Design review of the part built by this model. Coordinates are the model's own, in mm. Face numbers are marked on the shaded views. Coordinates: 2 decimals unless noted, no trailing zeros. Write each loop counter-clockwise with the first axis right and the second up, starting at its lowest first coordinate (ties: lowest second). Pieces come first, ordered by that corner, then holes. Notation, with made-up numbers: (-9, 72.25) - (11, 72.25) arc R14 cw to (11, 79.25) - close; hole circle Ø3 at (10, 35). An arc over 180 degrees is marked (long way). Answer as a JSON object with one key per item and string values.
```python
from build123d import *

# Parameters (mm, degrees)
EXTRUDE1_DEPTH = 2.286


with BuildPart() as part:
    # Sketch1 → Extrude1 (new body)
    with BuildSketch(Plane(origin=(0, 0, 0), x_dir=(1, 0, 0), z_dir=(0, 1, 0))):
        with BuildLine():
            Line((-35.587506478, 37.75591133), (35.587506478, 37.75591133))
            ThreePointArc((35.587506478, 37.75591133), (37.512064818, 37.331110288), (39.078987817, 36.135646762))
            Line((39.078987817, 36.135646762), (51.39211015, 21.570982059))
            ThreePointArc((51.39211015, 21.570982059), (52.406608959, 19.393408694), (52.177078973, 17.002101608))
            Line((52.177078973, 17.002101608), (36.497605157, -24.461395817))
            ThreePointArc((36.497605157, -24.461395817), (34.820154512, -26.605684768), (32.221154995, -27.416250797))
            Line((32.221154995, -27.416250797), (-32.221154995, -27.416250797))
            ThreePointArc((-32.221154995, -27.416250797), (-34.820154512, -26.605684768), (-36.497605157, -24.461395817))
            Line((-36.497605157, -24.461395817), (-52.177078973, 17.002101608))
            ThreePointArc((-52.177078973, 17.002101608), (-52.406608959, 19.393408694), (-51.39211015, 21.570982059))
            Line((-51.39211015, 21.570982059), (-39.078987817, 36.135646762))
            ThreePointArc((-39.078987817, 36.135646762), (-37.512064818, 37.331110288), (-35.587506478, 37.75591133))
        make_face()
    extrude(amount=-EXTRUDE1_DEPTH)


solid = part.part
```
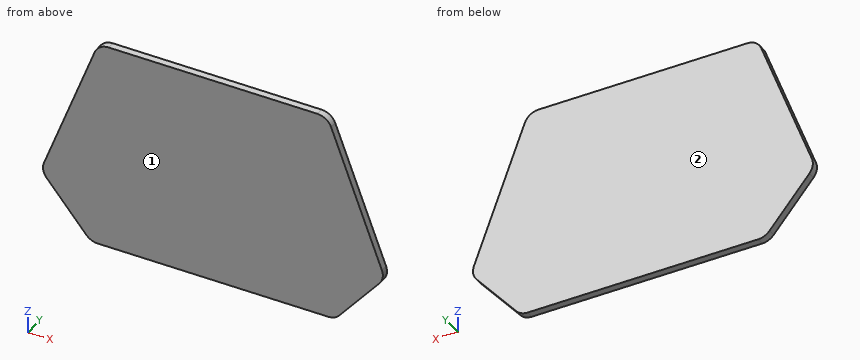
(1) Take a section at B-B, the plane z = 3. Write out the cut boundary in (x, y).
Solved:
{"outline": "(-44.61, -2.29) - (44.61, -2.29) - (44.61, 0) - (-44.61, 0) - close"}
(2) To check wall thickness, follow line 1 (Z direction, x = 32.5, y = -0.9); line 2 (X direction, y = -0.2, z = -17); line 3 (X direction, y = -1.3, z = -29.5). State the ranges of each line that lie inside material, in increasing order. Write a range as from..to.
Solved:
{"line 1": "z = -37.76..27.41", "line 2": "x = -52.18..52.18", "line 3": "x = -44.69..44.69"}
(3) Take a section at C-C, the plane z = -12.5. Write out the cut boundary in (x, y), and give its area (3 significant figures).
Solved:
{"outline": "(-50.47, -2.29) - (50.47, -2.29) - (50.47, 0) - (-50.47, 0) - close", "area": "231 mm^2"}
(4) Take a section at A-A, the plane y = -0.35. Write out the cut boundary in (x, z).
Solved:
{"outline": "(-52.18, -17) arc R4.57 ccw to (-51.39, -21.57) - (-39.08, -36.14) arc R4.57 ccw to (-35.59, -37.76) - (35.59, -37.76) arc R4.57 ccw to (39.08, -36.14) - (51.39, -21.57) arc R4.57 ccw to (52.18, -17) - (36.5, 24.46) arc R4.57 ccw to (32.22, 27.42) - (-32.22, 27.42) arc R4.57 ccw to (-36.5, 24.46) - close"}
(5) The part is to be moulded in two halves that separate along Y. For the marked faces 1 and 2, say which applies: pulls with the +Y half, pulls with the -Y half, needs draft (parallel to the pull), parting line crosses it, or undercut.
Solved:
{"face 1": "pulls with the -Y half", "face 2": "pulls with the +Y half"}
(6) For pin 1 (1 mm diameter, centred on y = -2, z = -7.5, fed in from +X), flat-tipped, find the tip position at first contact; note if it passes through.
Solved:
{"pin 1": "stops at x = 48.77"}
